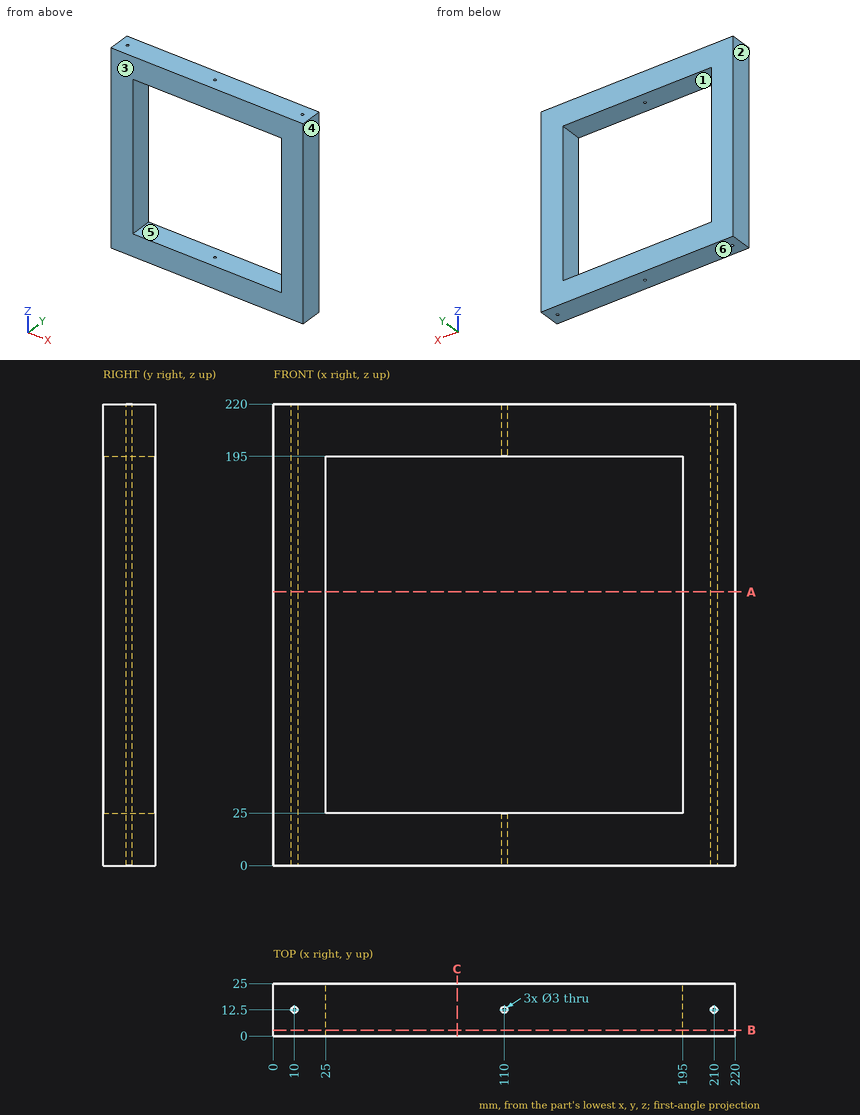
Check sheet for the drawn part. Datum: minimum x, y, z corner. Units: mm. A direction names the side the tool comes from. Give positions to 0.01 mm unless a question says otherwise; leave off trailing zeros. Order: outer loops, then holes, each group sorted by start corner. A loop starts at its lowest first (then second) coordinate and runs counter-clockwise, first axis right, second up. Notation, with made-up numbers: (57, 76) -> (65, 76) arc R21 cw to (65, 101) -> close; hole circle Ø7 at (44, -37). An arc over 180 degrees is marked (long way). Use a Markdown table: item, result.
1) Material ranges on probe 1 along X at (y, z) = (12.5, 46); probe 2 along X at (y, z) = (12.5, 215.25); probe 3 along Y at (x, z) = (10, 56.5), recorded low to high.
Results:
| item | result |
|---|---|
| probe 1 | 0 to 8.5, 11.5 to 25, 195 to 208.5, 211.5 to 220 |
| probe 2 | 0 to 8.5, 11.5 to 108.5, 111.5 to 208.5, 211.5 to 220 |
| probe 3 | 0 to 11, 14 to 25 |
2) Section check A-A, the plane z = 130.5. Record the boundary of the cut face in (x, y), then the cut area to 3 significant figures.
Results:
| item | result |
|---|---|
| outline | (0, 0) -> (25, 0) -> (25, 25) -> (0, 25) -> close; (195, 0) -> (220, 0) -> (220, 25) -> (195, 25) -> close; hole circle Ø3 at (10, 12.5); hole circle Ø3 at (210, 12.5) |
| area | 1,240 mm² |
3) Mould release check, pull along X, two halves, no side actions. Record for the marked faces 1, 2, 3 and 4: pulls with the +X half, pulls with the -X half, needs draft (parallel to the pull), parting line crosses it, or undercut.
Results:
| item | result |
|---|---|
| face 1 | undercut |
| face 2 | pulls with the -X half |
| face 3 | needs draft |
| face 4 | pulls with the +X half |
4) Section check B-B, the plane y = 2.75. Record the boundary of the cut face in (x, z), then the cut area to 3 significant figures.
Results:
| item | result |
|---|---|
| outline | (0, 0) -> (220, 0) -> (220, 220) -> (0, 220) -> close; hole (25, 25) -> (195, 25) -> (195, 195) -> (25, 195) -> close |
| area | 19,500 mm² |
5) Section check C-C, the plane x = 87.5. Record the boundary of the cut face in (y, z).
Results:
| item | result |
|---|---|
| outline | (0, 0) -> (25, 0) -> (25, 25) -> (0, 25) -> close; (0, 195) -> (25, 195) -> (25, 220) -> (0, 220) -> close |
6) Tool access check on the marked faces 5 and 6. Record the directions out of +Z, -Z, +X, -X, +Y, -Y that give a thin tool (end or side, any length) a straight path to the whole face; none if there is none.
Results:
| item | result |
|---|---|
| face 5 | +Y, -Y |
| face 6 | -Z, +X, -X, +Y, -Y |
